from build123d import *

# Parameters (mm, degrees)
BOSS_EXTRUDE2_DEPTH = 1.27
CUT_EXTRUDE1_DEPTH  = 100.076


with BuildPart() as part:
    # Sketch2 → Boss-Extrude2 (new, symmetric)
    with BuildSketch(Plane.XY):
        Polygon((-30.279813291, 84.630063366), (-78.379813291, 36.530063366), (-78.379813291, 0), (-27.5, 0), (-27.5, 84.630063366), align=None)
    extrude(amount=BOSS_EXTRUDE2_DEPTH, both=True)

    # Sketch3 → Cut-Extrude1 (cut)
    with BuildSketch(Plane(origin=(0, 0, 0), x_dir=(0, 0, -1), z_dir=(1, 0, 0))):
        Polygon((0, 84.630063366), (-1.27, 42.315031683), (-13.710908903, 42.315031683), (-13.710908903, 86.832104907), (21.305265315, 86.832104907), (21.305265315, 42.315031683), (1.27, 42.315031683), align=None)
    extrude(amount=-CUT_EXTRUDE1_DEPTH, mode=Mode.SUBTRACT)


solid = part.part
Could you check a few things on this model? Use its own coordinates, in mm. Give positions to 0.01 mm unless a question says otherwise; leave off trailing zeros. Order: outer loops, then holes, each group sorted by start corner. A loop starts at its lowest first (then second) coordinate and runs counter-clockwise, first axis right, second up.
Item 1: If we section it at C-C, the plane y = 77: Write out the boundary of the cut face in (x, z).
Item 2: If we section it at B-B, the plane z = -0.5: Write out the boundary of the cut face in (x, y), plus the area to 3 significant figures.
Item 3: If we section it at A-A, the plane x = -64: Write out the boundary of the cut face in (y, z), plus the area to 3 significant figures.
Item 4: If we section it at D-D, the plane x = -57: Write out the boundary of the cut face in (y, z).
Item 5: I need wall thicknesses on line 1 (Y direction, x = -58.5, z = 0.35); line 2 (Y direction, x = -75, z = -0.35); line 3 (X direction, y = 58, z = 0.1). Which ranges of each line are inside material? Lowest first, please.
Values:
1. outline: (-37.91, -0.23) - (-27.5, -0.23) - (-27.5, 0.23) - (-37.91, 0.23) - close
2. outline: (-78.38, 0) - (-27.5, 0) - (-27.5, 67.97) - (-46.94, 67.97) - (-78.38, 36.53) - close
2. area: 2,960 mm2
3. outline: (0, -1.27) - (42.32, -1.27) - (50.91, -1.01) - (50.91, 1.01) - (42.32, 1.27) - (0, 1.27) - close
3. area: 127 mm2
4. outline: (0, -1.27) - (42.32, -1.27) - (57.91, -0.8) - (57.91, 0.8) - (42.32, 1.27) - (0, 1.27) - close
5. line 1: y = 0 to 56.41
5. line 2: y = 0 to 39.91
5. line 3: x = -56.91 to -27.5
